Input: dimensioned drawing with shaded views. Units: mm. Origin: part minimum x, y, z. A direction names the side the tool comes from. Round coordinates to 2 decimals unless told otherwise and drop trailing zeros. Order: outer loops, then holes, each group sorted by start corner. A loop starts at its lowest first (then second) coordinate and runs counter-clockwise, first axis right, second up. Notation, with made-up numbers: M 7.5,-1 L 22.5,-1 A7 cw 22.5,12 Z; hole C 70,-6.75 d10. An arc over 180 degrees is marked long. Answer as CSV lines item,"result". Start each with the question number.
Item 1: Set-up query: the marked faces 1, 2 and 3. Return all of +Z, -Z, +X, -X, +Y, -Y with unobstructed straight access to the full face (end or side cutting, diameter ignored); none if empty.
Item 2: Section query A-A on z = 6.8. Return the cut outline in (x, y).
Item 3: Pull-direction query (X, two-part tool) for the marked faces 4, 5, 6 and 7; classes: +X half, -X half, draft (parallel to the pull), parting line (faces both ways), or undercut.
Item 4: Section query D-D on y = 7.5. Return the cut outline in (x, z).
Item 5: Line query: line 1 (X direction, y = 8.5, z = 19); line 2 (Z direction, x = 4.25, y = 4.5) (1 decimal); line 3 (X direction, y = 4.5, z = 6.8). Output: solid intervals per line, ascending. Write a range as [from, to].
Item 6: Section query C-C on x = 11.5. Return the cut outline in (y, z).
Item 7: First-contact query: P1, Ø4, axis at y = 7, z = 16.5, coming from the -X side; P2, Ø2, axis at y = 7, z = 12.5, coming from the +X side (1 decimal); P3, Ø6, axis at x = 5, z = 13, coming from the -Y side; P4, Ø6, axis at x = 3.5, y = 6.5, coming from the -Z side. Flat tips, straight axial feed; report the tip coordinate or a pass-through.
Item 8: Section query B-B on y = 5. Return the cut outline in (x, z).
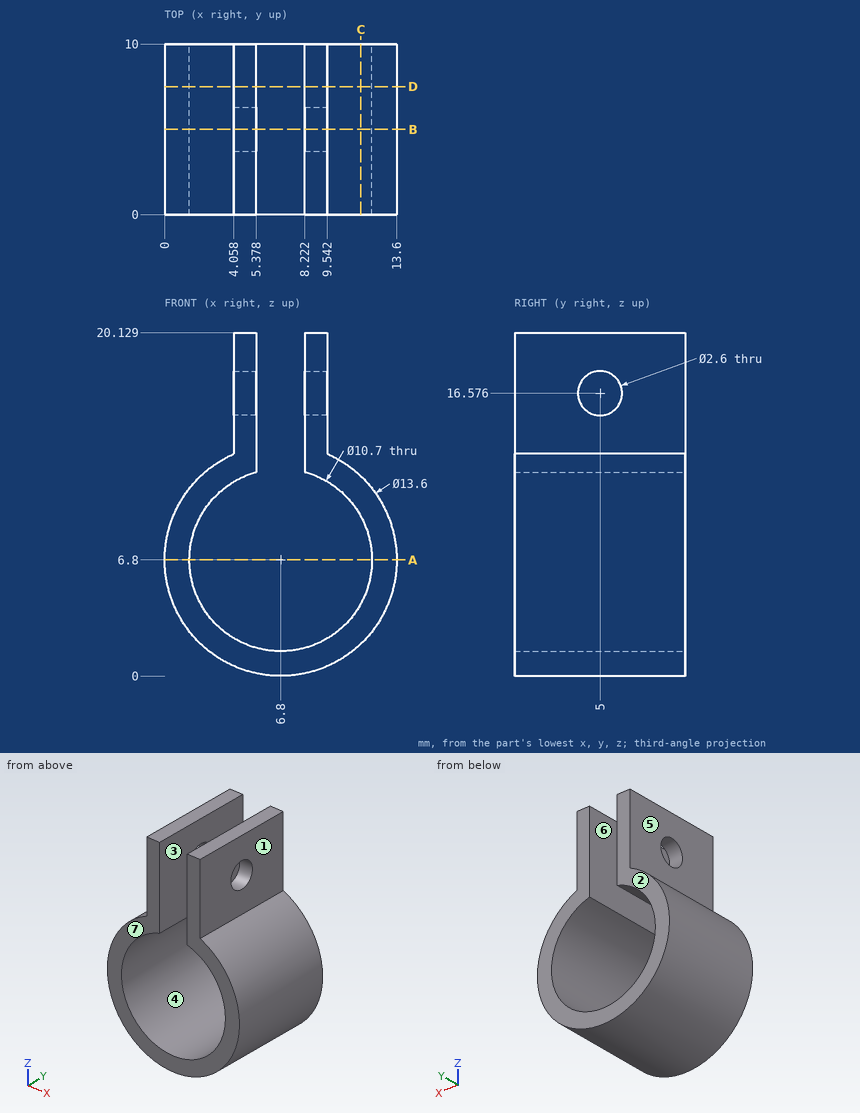
Results:
1,face 1,"+Z, +X, +Y, -Y"
1,face 2,"+Z, -Z, +X, -X, +Y"
1,face 3,"+Z, +Y, -Y"
2,outline,"M 0,0 L 1.45,0 L 1.45,10 L 0,10 Z; M 12.15,0 L 13.6,0 L 13.6,10 L 12.15,10 Z"
3,face 4,"undercut"
3,face 5,"-X half"
3,face 6,"undercut"
3,face 7,"draft"
4,outline,"M 4.06,13.02 A6.8 ccw long 9.54,13.02 L 9.54,20.13 L 8.22,20.13 L 8.22,11.96 A5.35 cw long 5.38,11.96 L 5.38,20.13 L 4.06,20.13 Z"
5,line 1,"[4.06, 5.38], [8.22, 9.54]"
5,line 2,"[0.5, 2.1], [11.5, 15.4], [17.8, 20.1]"
5,line 3,"[0, 1.45], [12.15, 13.6]"
6,outline,"M 0,1.89 L 10,1.89 L 10,4.24 L 0,4.24 Z; M 0,9.36 L 10,9.36 L 10,11.71 L 0,11.71 Z"
7,P1,"x = 4.06"
7,P2,"x = 11.7"
7,P3,"y = 0"
7,P4,"z = 0.01"
8,outline,"M 4.06,13.02 A6.8 ccw long 9.54,13.02 L 9.54,15.28 L 8.22,15.28 L 8.22,11.96 A5.35 cw long 5.38,11.96 L 5.38,15.28 L 4.06,15.28 Z; M 4.06,17.88 L 5.38,17.88 L 5.38,20.13 L 4.06,20.13 Z; M 8.22,17.88 L 9.54,17.88 L 9.54,20.13 L 8.22,20.13 Z"
